```python
from build123d import *

# Parameters (mm, degrees)
SKETCH1_R                = 66
BOSS_EXTRUDE1_DEPTH      = 7.5
SKETCH1_4_R              = 68
SKETCH1_4_R_2            = 66
BOSS_EXTRUDE3_DEPTH      = 2
BOSS_EXTRUDE4_START      = -2
SKETCH4_R                = 68
BOSS_EXTRUDE4_DEPTH      = 2
CUT_EXTRUDE1_DEPTH       = 97.458540317
CUT_EXTRUDE2_DEPTH       = 97.458540317
FILLET1_R                = 5
CIRPATTERN1_COUNT        = 6
FILLET1_OF_CIRPATTERN1_R = 5


with BuildPart() as part:
    # Sketch1 → Boss-Extrude1 (new body)
    with BuildSketch(Plane(origin=(0, 0, 0), x_dir=(1, 0, 0), z_dir=(0, 1, 0))):
        with Locations(Location((0, 0, 0), (0, 0, 270))):
            Circle(SKETCH1_R)
    extrude(amount=BOSS_EXTRUDE1_DEPTH)

    # Sketch1_4 → Boss-Extrude3 (add)
    with BuildSketch(Plane(origin=(0, 0, 0), x_dir=(1, 0, 0), z_dir=(0, 1, 0))):
        with Locations(Location((0, 0, 0), (0, 0, 270))):
            Circle(SKETCH1_4_R)
        with Locations(Location((0, 0, 0), (0, 0, 270))):
            Circle(SKETCH1_4_R_2, mode=Mode.SUBTRACT)
    extrude(amount=BOSS_EXTRUDE3_DEPTH)

    # Sketch4 → Boss-Extrude4 (add)
    with BuildSketch(Plane(origin=(0, 7.5, 0), x_dir=(1, 0, 0), z_dir=(0, 1, 0)).offset(BOSS_EXTRUDE4_START)):
        with Locations(Location((0, 0, 0), (0, 0, 270))):
            Circle(SKETCH4_R)
    extrude(amount=BOSS_EXTRUDE4_DEPTH)

    # Sketch6 → Cut-Extrude1 (cut, through all)
    with BuildSketch(Plane(origin=(0, 7.5, 0), x_dir=(1, 0, 0), z_dir=(0, 1, 0))):
        Polygon((-6.589092189, 3.594050285), (-6.407084944, -3.909296081), (0.182007245, -7.503346367), (6.589092189, -3.594050285), (6.407084944, 3.909296081), (-0.182007245, 7.503346367), align=None)
    extrude(amount=-CUT_EXTRUDE1_DEPTH, mode=Mode.SUBTRACT)

    # Sketch7 → Cut-Extrude2 (cut, through all)
    with BuildSketch(Plane(origin=(0, 7.5, 0), x_dir=(1, 0, 0), z_dir=(0, 1, 0))):
        with BuildLine():
            Line((-4.427257323, 7.255990118), (-48.322035968, 31.198596652))
            ThreePointArc((-48.322035968, 31.198596652), (-30.84284899, 50.549446572), (-5.639741154, 57.241286786))
            Line((-5.639741154, 57.241286786), (-4.427257323, 7.255990118))
        make_face()
    cut_extrude2 = extrude(amount=-CUT_EXTRUDE2_DEPTH, mode=Mode.SUBTRACT)

    # Fillet1
    fillet1_edges = [part.edges().sort_by_distance(p)[0] for p in [
        (-4.427257323, 3.75, -7.255990118),
        (-48.322035968, 3.75, -31.198596652),
        (-5.639741154, 3.75, -57.241286786),
    ]]
    fillet(fillet1_edges, radius=FILLET1_R)

    # CirPattern1: Cut-Extrude2 ×6 about axis
    cirpattern1_axis = Axis((0, 0, 0), (0, 1, 0))
    for i in range(1, CIRPATTERN1_COUNT):
        add(cut_extrude2.rotate(cirpattern1_axis, i * 360 / CIRPATTERN1_COUNT), mode=Mode.SUBTRACT)

    # Fillet1 of CirPattern1
    fillet1_of_cirpattern1_edges = [part.edges().sort_by_distance(p)[0] for p in [
        (-8.497500434, 3.75, 0.206122251),
        (-51.179795248, 3.75, 26.248812385),
        (-52.392279079, 3.75, -23.736484283),
        (-4.070243111, 3.75, 7.46211237),
        (-2.857759279, 3.75, 57.447409037),
        (-46.752537925, 3.75, 33.504802503),
        (4.427257323, 3.75, 7.255990118),
        (48.322035968, 3.75, 31.198596652),
        (5.639741154, 3.75, 57.241286786),
        (8.497500434, 3.75, -0.206122251),
        (51.179795248, 3.75, -26.248812385),
        (52.392279079, 3.75, 23.736484283),
        (4.070243111, 3.75, -7.46211237),
        (2.857759279, 3.75, -57.447409037),
        (46.752537925, 3.75, -33.504802503),
    ]]
    fillet(fillet1_of_cirpattern1_edges, radius=FILLET1_OF_CIRPATTERN1_R)


solid = part.part
```
Model file for the job. Use its own axes, mm. A direction names the side the tool comes from. Coordinates: 2 decimals unless noted, no trailing zeros. Order: outer loops, then holes, each group sorted by start corner. A loop starts at its lowest first (then second) coordinate and runs counter-clockwise, first axis right, second up. Notation, with made-up numbers: (63, 85) -> (76, 85) arc R16 ccw to (76, 101) -> close; hole circle Ø1 at (-3, 31.5). An arc over 180 degrees is marked (long way). Answer as a JSON object with one key per item and string values. Group by question number.
1) Cut at C-C, the plane x = -24.5. Write the cut outline in (y, z), then the cut area to 3 significant figures.
2) Cut at D-D, the plane y = 4. Count the separate pieces of the cut face and the enclosed holes in it, then the cut area to 3 significant figures.
3) Cut at A-A, the plane x = -50.5. Write the cut outline in (y, z), then the cut area to 3 significant figures.
4) Drill centre lines: L1, parallel to Z at x = 30, y = 6.75; L2, parallel to Z at x = 19, y = 4.25; L3, parallel to X at y = 3.75, z = 18.5. Where is each one in solid material? Low to high.
5) Which spindle directions (+Z, -Z, +X, -X, +Y, -Y) get a long thin tool onto all of the face, cutting with end or side? Do faces 5 (the face through (1, 0, 14)), 6 (the face through (3.16, 3.8, -5.68)). Say none if no direction does.
6) Flat gauge pin, fed straight in: pin 1 (1.5 mm diameter, centred on y = 3.5, z = -32, fed in from -X). Where does the tip first touch, or does it go through?
7) Cut at B-B, the plane z = 0. Write the cut outline in (x, y).
8) Pull direction Z, two halves, no side cores. Call faces 1 (the face through (7.141, 3.698, 55.794)), 2 (the face through (-64.43, 3.73, -14.31)), 3 (the face through (51.889, 3.698, 21.713)), 4 (the face through (1, 7.5, 14)): +Z half, -Z half, draft (parallel to the pull), parting line (faces both ways), or undercut.
Check values:
{
 "1": {"outline": "(0, -63.43) -> (2, -63.43) -> (2, -61.28) -> (5.5, -61.28) -> (5.5, -63.43) -> (7.5, -63.43) -> (7.5, -53.77) -> (0, -53.77) -> close; (0, -18.2) -> (7.5, -18.2) -> (7.5, -8.52) -> (0, -8.52) -> close; (0, 9.97) -> (7.5, 9.97) -> (7.5, 19.93) -> (0, 19.93) -> close; (0, 53.86) -> (7.5, 53.86) -> (7.5, 63.43) -> (5.5, 63.43) -> (5.5, 61.28) -> (2, 61.28) -> (2, 63.43) -> (0, 63.43) -> close", "area": "277 mm²"},
 "2": {"separate pieces": "1", "enclosed holes": "7", "area": "5,710 mm²"},
 "3": {"outline": "(0, -45.54) -> (2, -45.54) -> (2, -42.49) -> (5.5, -42.49) -> (5.5, -45.54) -> (7.5, -45.54) -> (7.5, -21.94) -> (0, -21.94) -> close; (0, 24.27) -> (7.5, 24.27) -> (7.5, 45.54) -> (5.5, 45.54) -> (5.5, 42.49) -> (2, 42.49) -> (2, 45.54) -> (0, 45.54) -> close", "area": "315 mm²"},
 "4": {"L1": "z = -61.02 to -51.04, -23.28 to -13.33, 11.52 to 21.2, 51.05 to 61.02", "L2": "z = -63.21 to -55.82, -16.57 to -6.61, 5.52 to 15.2, 55.65 to 63.21", "L3": "x = -63.35 to -55.46, -38.48 to -22.16, -3.8 to 4.7, 25.04 to 42.79, 55.17 to 63.35"},
 "5": {"face 5": "+Z, -Z, +X, -X, -Y", "face 6": "+Y, -Y"},
 "6": {"pin 1": "stops at x = -58.13"},
 "7": {"outline": "(-68, 0) -> (-59.21, 0) -> (-59.21, 7.5) -> (-68, 7.5) -> (-68, 5.5) -> (-66, 5.5) -> (-66, 2) -> (-68, 2) -> close; (-13.51, 0) -> (-6.5, 0) -> (-6.5, 7.5) -> (-13.51, 7.5) -> close; (6.5, 0) -> (13.51, 0) -> (13.51, 7.5) -> (6.5, 7.5) -> close; (59.21, 0) -> (68, 0) -> (68, 2) -> (66, 2) -> (66, 5.5) -> (68, 5.5) -> (68, 7.5) -> (59.21, 7.5) -> close"},
 "8": {"face 1": "undercut", "face 2": "parting line", "face 3": "undercut", "face 4": "draft"}
}
